from build123d import *

# Parameters (mm, degrees)
BOSS_EXTRUDE1_DEPTH = 6.5
SKETCH2_R           = 4
BOSS_EXTRUDE2_DEPTH = 40.8
CHAMFER1_SIZE       = 1


with BuildPart() as part:
    # Sketch1 → Boss-Extrude1 (new body)
    with BuildSketch(Plane.XY):
        with BuildLine():
            Line((28.196852764, -18.321256673), (29, -17.010639502))
            ThreePointArc((29, -17.010639502), (17.75919782, -5.237578059), (4.294710806, 3.909454184))
            ThreePointArc((4.294710806, 3.909454184), (-13.701993595, 7.383969683), (-30.515502146, 0.086055087))
            ThreePointArc((-30.515502146, 0.086055087), (-31.755615747, -1.187280745), (-32.750708825, -2.660052163))
            ThreePointArc((-32.750708825, -2.660052163), (-32.488602214, -6.256255028), (-29.091806444, -7.465863814))
            ThreePointArc((-29.091806444, -7.465863814), (0.718290474, -6.741295906), (28.196852764, -18.321256673))
        make_face()
    extrude(amount=BOSS_EXTRUDE1_DEPTH)

    # Sketch2 → Boss-Extrude2 (add)
    with BuildSketch(Plane(origin=(0, 0, 0), x_dir=(-1, 0, 0), z_dir=(0, 0, -1))):
        Circle(SKETCH2_R)
    extrude(amount=BOSS_EXTRUDE2_DEPTH)

    # Chamfer1
    chamfer1_edges = [part.edges().sort_by_distance(p)[0] for p in [
        (4, 0, -40.8),
    ]]
    chamfer(chamfer1_edges, length=CHAMFER1_SIZE)


solid = part.part
The model under review builds one solid part; all positions refer to its coordinate system, in mm. Give positions to 0.01 mm unless a question says otherwise; leave off trailing zeros. Order: outer loops, then holes, each group sorted by start corner. A loop starts at its lowest first (then second) coordinate and runs counter-clockwise, first axis right, second up. Notation, with made-up numbers: M -16.75,50.25 L 36.25,50.25 A32 cw 36.25,76.25 Z; hole C 42.5,67 d9. An arc over 180 degrees is marked long. Answer in a Markdown table with one row per item. Add a question column.
1. For pin 1 Ø6 at (y, z) = (-4.5, -12.5) entering from +X; pin 2 Ø10 at (y, z) = (-1.5, -12) entering from +X; pin 3 Ø6 at (x, y) = (12, -8.5) entering from -Z; pin 4 Ø4 at (x, y) = (-2.5, -10) entering from +Z, all flat-tipped, find the tip position at first contact; note any pin that passes through.
2. Add section C-C on y = -13.5. State the section outline as (x, z) points.
3. Mouldability with a two-part tool opening along X and no side actions: class faces 1 (the cylindrical face through (0.305, -6.664, 3.204)), 2 (the cylindrical face through (0.867, -3.905, -19.621)), 3 (the flat face through (-5, -2, 0)) as released by +X, released by -X, zero draft, split by the parting line, or undercut.
4. Add section A-A on z = -27. State the section outline as (x, y) points, plus the area to 3 significant figures.
5. Add section B-B on x = 0. State the section outline as (y, z) points.
6. To check wall thickness, follow line 1 along Z through (x, y) = (7.5, -2.25); line 2 along Y through (x, z) = (-0.5, 4.5); line 3 along Y through (x, z) = (2.5, -12.5). State the ranges of each line that lie inside material, in increasing order.
7. Add section D-D on x = -18. State the section outline as (y, z) points.
The answers:
| question | item | result |
|---|---|---|
| 1 | pin 1 | x = 3.71 |
| 1 | pin 2 | x = 4 |
| 1 | pin 3 | z = 0 |
| 1 | pin 4 | through |
| 2 | outline | M 20.24,0 L 26.13,0 L 26.13,6.5 L 20.24,6.5 Z |
| 3 | face 1 | undercut |
| 3 | face 2 | split by the parting line |
| 3 | face 3 | zero draft |
| 4 | outline | C 0,0 d8 |
| 4 | area | 50.3 mm2 |
| 5 | outline | M -6.61,0 L -4,0 L -4,-39.8 L -3,-40.8 L 3,-40.8 L 4,-39.8 L 4,0 L 5.8,0 L 5.8,6.5 L -6.61,6.5 Z |
| 6 | line 1 | 0 to 6.5 |
| 6 | line 2 | -6.52 to 5.97 |
| 6 | line 3 | -3.12 to 3.12 |
| 7 | outline | M -5.71,0 L 6.6,0 L 6.6,6.5 L -5.71,6.5 Z |
